from build123d import *

# Parameters (mm, degrees)
EXTRUDE_1_DEPTH = 30
SHELL_START     = 5
SHELL_1_DEPTH   = 25


# Read off the part's stored shape, not the designer's step: 薄殼1
with BuildPart() as part:
    # 草圖1 → 伸長1 (new body)
    with BuildSketch(Plane(origin=(0, 0, 0), x_dir=(1, 0, 0), z_dir=(0, 1, 0))):
        Polygon((0, 28.867513459), (-25, 14.43375673), (-25, -14.43375673), (0, -28.867513459), (25, -14.43375673), (25, 14.43375673), align=None)
    extrude(amount=EXTRUDE_1_DEPTH)

    # 薄殼1 outline → 薄殼1 (cut)
    with BuildSketch(Plane(origin=(0, 0, 0), x_dir=(1, 0, 0), z_dir=(0, 1, 0)).offset(SHELL_START)):
        Polygon((17, 13.279056191), (0, 23.094010768), (-20, 11.547005384), (-20, -11.547005384), (0, -23.094010768), (17, -13.279056191), align=None)
    extrude(amount=SHELL_1_DEPTH, mode=Mode.SUBTRACT)


solid = part.part
Input: part model. Units: mm. Frame: model coordinates. A direction names the side the tool comes from. Coordinates: 2 decimals unless noted, no trailing zeros. Loops run counter-clockwise (first coordinate to the right, second up) from the corner with the lowest first, then second, coordinate; pieces in that order, holes last.
Q1. Contact query for flat-ended pins moving along their axis: pin 1 (1 mm diameter, centred on x = -12.5, y = 16, fed in from +Z); pin 2 (1.5 mm diameter, centred on x = -12, y = 9, fed in from +Z); pin 3 (5 mm diameter, centred on x = 5.5, z = 14, fed in from +Y). Output: stop coordinate, or through.
Q2. Cut plane B-B (x = -4.5). Output: boundary loops of the cut face in (y, z), then the cut area to 3 significant figures.
Q3. Cut plane C-C (z = 18.5). Output: boundary loops of the cut face in (x, y).
Q4. Cut plane D-D (x = 22). Output: boundary loops of the cut face in (y, z).
Q5. Material intervals for line 1 (X direction, y = 12, z = -9.5); line 2 (Z direction, x = 0, y = 18.5); line 3 (Y direction, x = -6, z = 19), sorted ascending.
Q6. Cut plane A-A (y = 21.25). Output: boundary loops of the cut face in (x, z).
Q7. Draft query along Z for faces 1 (the face through (0, 0, 0)), 2 (the face through (-9.86, 17.32, -17.4)), 3 (the face through (12.675, 14.79, -21.55)). Return one class per face: +Z half, -Z half, draft (parallel to the pull), parting line (faces both ways), or undercut.
Q8. Set-up query: faces 4 (the face through (12.33, 14.79, 21.75)), 5 (the face through (17, 17, 0)). Return all of +Z, -Z, +X, -X, +Y, -Y with unobstructed straight access to the full face (end or side cutting, diameter ignored); none if empty.
Working result:
1. pin 1: stops at z = 21.94
1. pin 2: stops at z = 22.37
1. pin 3: stops at y = 5
2. outline: (0, -26.27) - (30, -26.27) - (30, -20.5) - (5, -20.5) - (5, 20.5) - (30, 20.5) - (30, 26.27) - (0, 26.27) - close
2. area: 551 mm2
3. outline: (-17.96, 0) - (17.96, 0) - (17.96, 30) - (7.96, 30) - (7.96, 5) - (-7.96, 5) - (-7.96, 30) - (-17.96, 30) - close
4. outline: (0, -16.17) - (30, -16.17) - (30, 16.17) - (0, 16.17) - close
5. line 1: x = -25 to -20, 17 to 25
5. line 2: z = -28.87 to -23.09, 23.09 to 28.87
5. line 3: y = 0 to 5
6. outline: (-25, -14.43) - (0, -28.87) - (25, -14.43) - (25, 14.43) - (0, 28.87) - (-25, 14.43) - close; hole (-20, -11.55) - (0, -23.09) - (17, -13.28) - (17, 13.28) - (0, 23.09) - (-20, 11.55) - close
7. face 1: draft
7. face 2: undercut
7. face 3: -Z half
8. face 4: +Z, +X, +Y, -Y
8. face 5: +Y
